The model under review builds one solid part; all positions refer to its coordinate system, in mm. A direction names the side the tool comes from. Round coordinates to 2 decimals unless told otherwise and drop trailing zeros. Write each loop counter-clockwise with the first axis right and the second up, starting at its lowest first coordinate (ties: lowest second). Pieces come first, ordered by that corner, then holes. Notation, with made-up numbers: M 76.5,75.5 L 91.5,75.5 A21 cw 91.5,113.5 Z; hole C 57.25,81 d7. An arc over 180 degrees is marked long. Write item = value, one per line. Start each with the question number.
Item 1: For pin 1 Ø3 at (y, z) = (32.5, 1.5) entering from -X; pin 2 Ø3 at (x, z) = (26.5, 0.5) entering from +Y; pin 3 Ø9 at (x, y) = (29, 8) entering from +Z; pin 4 Ø4 at (x, z) = (50, 1) entering from -Y, all flat-tipped, find the tip position at first contact; note any pin that passes through.
Item 2: Take a section at D-D, the plane x = 20.5. Give the boundary of the cut face in (y, z), plus the area to 3 significant figures.
Item 3: To check wall thickness, follow line 1 along Z through (x, y) = (34.5, 4); line 2 along X through (y, z) = (47, -0.5); line 3 along Y through (x, z) = (36, 0.75). State the ranges of each line that lie inside material, in increasing order.
Item 4: The part is to be moulded in two halves that separate along X. For faces 1 (the flat face through (0, 62.5, 0)), 2 (the flat face through (28, 11, 0)), say which applies: +X half, -X half, draft (parallel to the pull), parting line (faces both ways), or undercut.
Item 5: Take a section at B-B, the plane y = 37.5. Give the boundary of the cut face in (x, z).
Item 6: Tool access review of faces 3 (the flat face through (28, 0, 0)), 4 (the flat face through (56, 56, 0)), 5 (the flat face through (3, 54.5, 3)): name each direction out of +Z, -Z, +X, -X, +Y, -Y from which nothing blocks a thin tool from reaching the whole face with its end or side.
Item 7: Take a section at A-A, the plane z = 0. Give the boundary of the cut face in (x, y).
Item 8: Take a section at C-C, the plane x = 0. Give the boundary of the cut face in (y, z).
Autodesk Inventor part; units mm, degrees
ref_plane "YZ Plane" through (0, 0, 0) normal (1, 0, 0) x (0, 1, 0)
ref_plane "XZ Plane" through (0, 0, 0) normal (0, 1, 0) x (-1, 0, 0)
ref_plane "XY Plane" through (0, 0, 0) normal (0, 0, 1) x (1, 0, 0)
sketch "Sketch1" plane through (0, 0, 0) normal (0, 1, 0) x (-1, 0, 0)
  circle A0 centre (0, 0) radius 4
  dimension "d0" = 8
extrude "Extrusion1" add sketch "Sketch1" along normal blind 54.5
sketch "Sketch2" plane through (0, 54.5, 0) normal (0, 1, 0) x (1, 0, 0)
  circle A0 centre (0, 0) radius 7
  dimension "d3" = 14
extrude "Extrusion2" add sketch "Sketch2" along normal blind 8
sketch "Sketch3" plane through (0, 0, 0) normal (0, 0, 1) x (1, 0, 0)
  line L0 (0, 0) -> (56, 0)
  line L1 (56, 0) -> (56, 11)
  line L2 (56, 11) -> (0, 11)
  line L3 (0, 11) -> (0, 0)
  dimension "d6" = 56
  dimension "d7" = 11
extrude "Extrusion3" add sketch "Sketch3" along normal mid plane 3.5
sketch "Sketch12" plane through (0, 0, 0) normal (0, -1, 0) x (1, 0, 0)
  line L0 (56, 1.75) -> (56, -1.75)
  circle A0 centre (56, 0) radius 4
  line L1 (-20.4, 0) -> (73.4, 0)
  point P0 (0, 0)
  dimension "d41" = 8
extrude "Extrusion10" add sketch "Sketch12" against normal blind 56
properties part number "Cube Cage" material "ABS Plastic"
Response values:
q1.pin_1 = -4
q1.pin_2 = 11
q1.pin_3 = 1.75
q1.pin_4 = 0
q2.outline = M 0,-1.75 L 11,-1.75 L 11,1.75 L 0,1.75 Z
q2.area = 38.5 mm2
q3.line_1 = -1.75 to 1.75
q3.line_2 = -3.97 to 3.97, 52.03 to 59.97
q3.line_3 = 0 to 11
q4.face_1 = draft
q4.face_2 = undercut
q5.outline = C 0,0 d8; C 56,0 d8
q6.face_3 = +Z, -Z, +X, -X, -Y
q6.face_4 = +Z, -Z, +X, +Y
q6.face_5 = none
q7.outline = M -7,54.5 L -4,54.5 L -4,0 L 60,0 L 60,56 L 52,56 L 52,11 L 4,11 L 4,54.5 L 7,54.5 L 7,62.5 L -7,62.5 Z
q8.outline = M 0,-4 L 54.5,-4 L 54.5,-7 L 62.5,-7 L 62.5,7 L 54.5,7 L 54.5,4 L 0,4 Z
